For this review, take the finished solid that the model builds, in its own axes (mm). A direction names the side the tool comes from. Give positions to 0.01 mm unless a question says otherwise; leave off trailing zeros. Order: outer loops, then holes, each group sorted by start corner. A loop starts at its lowest first (then second) coordinate and runs counter-clockwise, first axis right, second up.
from build123d import *

# Parameters (mm, degrees)
F0_R      = 22.5
F0_R_2    = 8.1
F1_DEPTH  = 2.7
F2_R      = 2.4
F3_DEPTH  = 6.3
F4_R      = 3
F5_DEPTH  = 6.8
F6_R      = 1.95
F7_R      = 1.95
F8_R      = 1.95
F9_DEPTH  = 2
F10_R     = 19.95
F10_R_2   = 19.05
F11_DEPTH = 0.8


with BuildPart() as f1:
    # F0 (on Front) → F1 (new body)
    with BuildSketch(Plane.XZ):
        Circle(F0_R)
        Circle(F0_R_2, mode=Mode.SUBTRACT)
    extrude(amount=F1_DEPTH)

    # F2 (on face) → F3 (join)
    with BuildSketch(Plane.XZ.offset(2.7)):
        with Locations((0, 13.65)):
            Circle(F2_R)
        with Locations((-11.821247, -6.825)):
            Circle(F2_R)
        with Locations((11.821247, -6.825)):
            Circle(F2_R)
    extrude(amount=F3_DEPTH)

    # F4 (on face) → F5 (join)
    with BuildSketch(Plane.XZ.offset(2.7)):
        with Locations((0, -17.5)):
            Circle(F4_R)
        with Locations((15.155445, 8.75)):
            Circle(F4_R)
        with Locations((-15.155445, 8.75)):
            Circle(F4_R)
    extrude(amount=F5_DEPTH)

    # F6 (on face) + F7 (on face) + F8 (on face) → F9 (join)
    with BuildSketch(Plane.XZ.offset(9.5)):
        with Locations((0, -17.5)):
            Circle(F6_R)
    with BuildSketch(Plane.XZ.offset(9.5)):
        with Locations((-15.155445, 8.75)):
            Circle(F7_R)
    with BuildSketch(Plane.XZ.offset(9.5)):
        with Locations((15.155445, 8.75)):
            Circle(F8_R)
    extrude(amount=F9_DEPTH)

    # F10 (on face) → F11 (join)
    with BuildSketch(Plane(origin=(0, 0, 0), x_dir=(-1, 0, 0), z_dir=(0, 1, 0))):
        Circle(F10_R)
        Circle(F10_R_2, mode=Mode.SUBTRACT)
    extrude(amount=F11_DEPTH)


solid = f1.part
1) We need section A-A on z = 0. Give the boundary of the cut face in (x, y), then the cut area to 3 significant figures.
Answer sheet:
outline: (-22.5, -2.7) - (-8.1, -2.7) - (-8.1, 0) - (-19.05, 0) - (-19.05, 0.8) - (-19.95, 0.8) - (-19.95, 0) - (-22.5, 0) - close; (8.1, -2.7) - (22.5, -2.7) - (22.5, 0) - (19.95, 0) - (19.95, 0.8) - (19.05, 0.8) - (19.05, 0) - (8.1, 0) - close
area: 79.2 mm2
2) To check wall thickness, follow line 1 (Z direction, x = 0, y = -1.85); line 2 (Y direction, x = -2.5, z = 16); line 3 (X direction, y = -7.75, z = 7.5). State the ranges of each line that lie inside material, in increasing order.
Answer sheet:
line 1: z = -22.5 to -8.1, 8.1 to 22.5
line 2: y = -2.7 to 0
line 3: x = -17.88 to -12.43, 12.43 to 17.88
3) We need section B-B on x = 0. Give the boundary of the cut face in (y, z), then the cut area to 3 significant figures.
Answer sheet:
outline: (-11.5, -19.45) - (-9.5, -19.45) - (-9.5, -20.5) - (-2.7, -20.5) - (-2.7, -22.5) - (0, -22.5) - (0, -19.95) - (0.8, -19.95) - (0.8, -19.05) - (0, -19.05) - (0, -8.1) - (-2.7, -8.1) - (-2.7, -14.5) - (-9.5, -14.5) - (-9.5, -15.55) - (-11.5, -15.55) - close; (-9, 11.25) - (-2.7, 11.25) - (-2.7, 8.1) - (0, 8.1) - (0, 19.05) - (0.8, 19.05) - (0.8, 19.95) - (0, 19.95) - (0, 22.5) - (-2.7, 22.5) - (-2.7, 16.05) - (-9, 16.05) - close
area: 158 mm2
4) We need section C-C on x = -16. Give the boundary of the cut face in (y, z).
Answer sheet:
outline: (-11.5, 6.99) - (-9.5, 6.99) - (-9.5, 5.87) - (-2.7, 5.87) - (-2.7, -15.82) - (0, -15.82) - (0, -11.92) - (0.8, -11.92) - (0.8, -10.34) - (0, -10.34) - (0, 10.34) - (0.8, 10.34) - (0.8, 11.92) - (0, 11.92) - (0, 15.82) - (-2.7, 15.82) - (-2.7, 11.63) - (-9.5, 11.63) - (-9.5, 10.51) - (-11.5, 10.51) - close
5) Tool access review of faces 1 (the face through (15.12, 0.39, -11.59)), 2 (the face through (12, -9, -7)), 3 (the face through (-13.295, -10.486, 9.336)), 4 (the face through (10.382, -1.331, -19.961)): name each direction out of +Z, -Z, +X, -X, +Y, -Y from which nothing blocks a thin tool from reaching the whole face with its end or side.
Answer sheet:
face 1: +Y
face 2: -Z, +X, -X, -Y
face 3: -Y
face 4: +Y, -Y
6) We need section D-D on z = 13.65. Give the boundary of the cut face in (x, y).
Answer sheet:
outline: (-17.89, -2.7) - (-2.4, -2.7) - (-2.4, -9) - (2.4, -9) - (2.4, -2.7) - (17.89, -2.7) - (17.89, 0) - (14.55, 0) - (14.55, 0.8) - (13.29, 0.8) - (13.29, 0) - (-13.29, 0) - (-13.29, 0.8) - (-14.55, 0.8) - (-14.55, 0) - (-17.89, 0) - close
7) Draft analysis for pull direction X (two halves, no side actions). For faces 5 (the face through (0, -2.7, -10)), 6 (the face through (0.9, -10.49, -19.23)), 7 (the face through (15, -11.5, 9)), state which applies: +X half, -X half, draft (parallel to the pull), parting line (faces both ways), or undercut.
Answer sheet:
face 5: undercut
face 6: parting line
face 7: draft
8) Clearance check with flat-ended pins moving along their axes: pin 1 (4 mm diameter, centred on y = -6.5, z = 4.5, fed in from -X); pin 2 (12 mm diameter, centred on x = 5, z = -12.5, fed in from +Y); pin 3 (1.5 mm diameter, centred on x = 0.5, y = -1.5, fed in from -Z); pin 4 (4 mm diameter, centred on x = 13, z = -5.5, fed in from -Y). State where each tip first meets the part, or that it passes through.
Answer sheet:
pin 1: stops at x = -17.14
pin 2: stops at y = 0.8
pin 3: stops at z = -22.5
pin 4: stops at y = -9
